Design review of the part built by this model. Coordinates are the model's own, in mm. Coordinates: 2 decimals unless noted, no trailing zeros. Write each loop counter-clockwise with the first axis right and the second up, starting at its lowest first coordinate (ties: lowest second). Pieces come first, ordered by that corner, then holes.
Q1. For L1, parallel to Y at x = 312, z = 303.6; L2, parallel to Y at x = 346, z = 302.65; L3, parallel to Y at x = 349.5, z = 300.85, list the stretches that pass through material, from the lowest coordinate up.
Q2. Take a section at B-B, the plane x = 328. Write out the cut boundary in (y, z), plus the area to 3 significant figures.
Q3. Take a section at A-A, the plane x = 369. Write out the cut boundary in (y, z) (3 decimals).
Q4. For pin 1 Ø17.5 at (x, y) = (350, 315) entering from +Z, flat-tipped, find the tip position at first contact; note if it passes through.
Q5. Take a section at C-C, the plane z = 303.35. State how many separate pieces and enclosed holes the cut face has, plus the area to 3 significant figures.
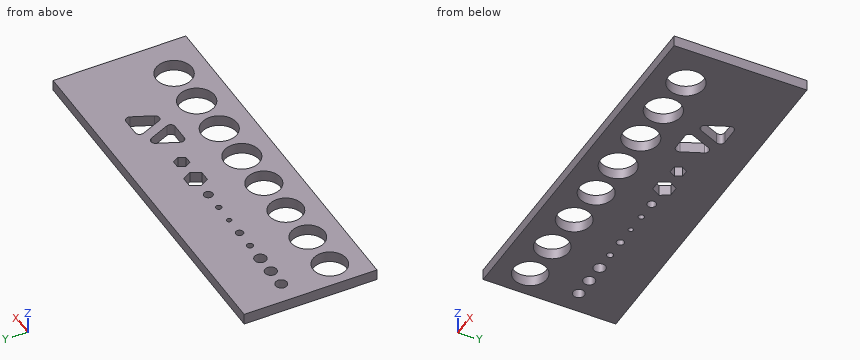
from build123d import *

# Parameters (mm, degrees)
SKETCH1_W           = 165
SKETCH1_H           = 60
SKETCH1_R           = 7.55
SKETCH1_R_2         = 7.575
SKETCH1_R_3         = 7.6
SKETCH1_R_4         = 7.625
SKETCH1_R_5         = 8.025
SKETCH1_R_6         = 8.05
SKETCH1_R_7         = 8.075
SKETCH1_R_8         = 8.1
SKETCH1_R_9         = 2.6
SKETCH1_R_10        = 2.65
SKETCH1_R_11        = 2.7
SKETCH1_R_12        = 1.45
SKETCH1_R_13        = 1.7
SKETCH1_R_14        = 1.1
SKETCH1_R_15        = 1.3
SKETCH1_R_16        = 2
BOSS_EXTRUDE1_DEPTH = 5


with BuildPart() as part:
    # Sketch1 → Boss-Extrude1 (new body)
    with BuildSketch(Plane.XY.offset(300)):
        with Locations((382.5, 330)):
            Rectangle(SKETCH1_W, SKETCH1_H)
        with Locations((312, 315)):
            Circle(SKETCH1_R, mode=Mode.SUBTRACT)
        with Locations((331, 315)):
            Circle(SKETCH1_R_2, mode=Mode.SUBTRACT)
        with Locations((350, 315)):
            Circle(SKETCH1_R_3, mode=Mode.SUBTRACT)
        with Locations((369, 315)):
            Circle(SKETCH1_R_4, mode=Mode.SUBTRACT)
        with Locations((388, 315)):
            Circle(SKETCH1_R_5, mode=Mode.SUBTRACT)
        with Locations((407.5, 315)):
            Circle(SKETCH1_R_6, mode=Mode.SUBTRACT)
        with Locations((427, 315)):
            Circle(SKETCH1_R_7, mode=Mode.SUBTRACT)
        with Locations((446.5, 315)):
            Circle(SKETCH1_R_8, mode=Mode.SUBTRACT)
        with Locations((310, 338)):
            Circle(SKETCH1_R_9, mode=Mode.SUBTRACT)
        with Locations((319, 338)):
            Circle(SKETCH1_R_10, mode=Mode.SUBTRACT)
        with Locations((328, 338)):
            Circle(SKETCH1_R_11, mode=Mode.SUBTRACT)
        with Locations((337, 338)):
            Circle(SKETCH1_R_12, mode=Mode.SUBTRACT)
        with Locations((346, 338)):
            Circle(SKETCH1_R_13, mode=Mode.SUBTRACT)
        with Locations((355, 338)):
            Circle(SKETCH1_R_14, mode=Mode.SUBTRACT)
        with Locations((364, 338)):
            Circle(SKETCH1_R_15, mode=Mode.SUBTRACT)
        with Locations((373, 338)):
            Circle(SKETCH1_R_16, mode=Mode.SUBTRACT)
        Polygon((388.734272207, 338), (386.367136104, 342.1), (381.632863896, 342.1), (379.265727793, 338), (381.632863896, 333.9), (386.367136104, 333.9), align=None, mode=Mode.SUBTRACT)
        Polygon((399.290896534, 338), (397.645448267, 340.85), (394.354551733, 340.85), (392.709103466, 338), (394.354551733, 335.15), (397.645448267, 335.15), align=None, mode=Mode.SUBTRACT)
        with BuildLine():
            Line((409.05803115, 330), (416.94196885, 330))
            ThreePointArc((416.94196885, 330), (418.615778179, 330.90530263), (418.77428352, 332.801637668))
            Line((418.77428352, 332.801637668), (414.83231467, 341.811852183))
            ThreePointArc((414.83231467, 341.811852183), (413, 343.010214515), (411.16768533, 341.811852183))
            Line((411.16768533, 341.811852183), (407.22571648, 332.801637668))
            ThreePointArc((407.22571648, 332.801637668), (407.384221821, 330.90530263), (409.05803115, 330))
        make_face(mode=Mode.SUBTRACT)
        with BuildLine():
            Line((426.63231467, 334.188147817), (430.57428352, 343.198362332))
            ThreePointArc((430.57428352, 343.198362332), (430.415778179, 345.09469737), (428.74196885, 346))
            Line((428.74196885, 346), (420.85803115, 346))
            ThreePointArc((420.85803115, 346), (419.184221821, 345.09469737), (419.02571648, 343.198362332))
            Line((419.02571648, 343.198362332), (422.96768533, 334.188147817))
            ThreePointArc((422.96768533, 334.188147817), (424.8, 332.989785485), (426.63231467, 334.188147817))
        make_face(mode=Mode.SUBTRACT)
    extrude(amount=BOSS_EXTRUDE1_DEPTH)


solid = part.part
Responses:
1. L1: y = 300 to 307.45, 322.55 to 336.34, 339.66 to 360
1. L2: y = 300 to 308.54, 321.46 to 336.3, 339.7 to 360
1. L3: y = 300 to 307.42, 322.58 to 360
2. outline: (300, 300) - (308.04, 300) - (308.04, 305) - (300, 305) - close; (321.96, 300) - (335.3, 300) - (335.3, 305) - (321.96, 305) - close; (340.7, 300) - (360, 300) - (360, 305) - (340.7, 305) - close
2. area: 203 mm2
3. outline: (300, 300) - (307.375, 300) - (307.375, 305) - (300, 305) - close; (322.625, 300) - (360, 300) - (360, 305) - (322.625, 305) - close
4. pin 1: stops at z = 305
5. separate pieces: 1
5. enclosed holes: 20
5. area: 7,960 mm2
